Work out the finished part from the listing and answer in its coordinate system (mm). Give positions to 0.01 mm unless a question says otherwise; leave off trailing zeros. Loops run counter-clockwise (first coordinate to the right, second up) from the corner with the lowest first, then second, coordinate; pieces in that order, holes last. Notation, with made-up numbers: (28, -2) - (82, -2) arc R14 cw to (82, 24) - close; hole circle Ø7 at (-12.75, -20.75). An arc over 180 degrees is marked (long way). One line per question, with ' | ' between items. Start each with the question number.
1. Section C-C (y = -5.25) is taken. Determine the outline of the cut face in (x, z), plus the area to 3 significant figures.
2. Section A-A (x = 68) is taken. Determine the outline of the cut face in (y, z), plus the area to 3 significant figures.
3. Find the intervals of material crossed by line 1 (X direction, y = -10.25, z = 318.5); line 2 (Z direction, x = 124, y = -7); line 3 (Z direction, x = 54, y = -14), in increasing order.
4. Section B-B (z = 82) is taken. Determine the outline of the cut face in (x, y), plus the area to 3 significant figures.
from build123d import *

# Parameters (mm, degrees)
F0_W      = 28.8499742746
F0_H      = 37.8827601671
F1_DEPTH  = 16
F2_DEPTH  = 296
F3_DEPTH  = 996
F4_W      = 199.8313069344
F4_H      = 801.1276721954
F5_DEPTH  = 5
F6_DEPTH  = 39.21
F7_DEPTH  = 2.24
F8_DEPTH  = 55.66
F9_DEPTH  = 1.59
F10_W     = 54.77245152
F10_H     = 895.9976721954
F11_DEPTH = 5
F12_DEPTH = 5.86
F13_DEPTH = 18.91
F14_W     = 83.0026693535
F14_H     = 34.9487662315
F14_H_2   = 55.274695158
F15_W     = 82.9961860609
F15_H     = 44.8832511902
F15_H_2   = 52.5203943253
F16_DEPTH = 5
F17_DEPTH = 300
F18_DEPTH = 300
F19_DEPTH = 324.79
F20_DEPTH = 324.79
F21_DEPTH = 250
F22_DEPTH = 250
F23_DEPTH = 100
F24_DEPTH = 100
F25_DEPTH = 50
F26_DEPTH = 50
F27_DEPTH = 134.02
F28_DEPTH = 100
F29_DEPTH = 100
F30_DEPTH = 100
F31_DEPTH = 50
F32_DEPTH = 54.95
F33_DEPTH = 50
F34_DEPTH = 109.29
F35_DEPTH = 14.88
F36_DEPTH = 230.15
F37_DEPTH = 230.15
F38_DEPTH = 22.52
F39_DEPTH = 77.2
F40_DEPTH = 77.2
F41_DEPTH = 11
F42_R     = 3


with BuildPart() as f1:
    # F0 (on Front) → F1 (new body)
    with BuildSketch(Plane.XZ):
        with Locations((14.4249871373, 18.9413800836)):
            Rectangle(F0_W, F0_H)
    extrude(amount=F1_DEPTH)

    # F2 (add): a face of the model
    f2_faces = [f1.faces().sort_by_distance(p)[0] for p in [
        (0, -8, 18.9413800836),
    ]]
    extrude(f2_faces, amount=-F2_DEPTH)

    # F3 (add): a face of the model
    f3_faces = [f1.faces().sort_by_distance(p)[0] for p in [
        (148, -8, 0),
    ]]
    extrude(f3_faces, amount=-F3_DEPTH)

    # F4 (on face) → F5 (cut)
    with BuildSketch(Plane.XZ.offset(16)):
        with Locations((148.3252942562, 506.2239170074)):
            Rectangle(F4_W, F4_H)
    extrude(amount=-F5_DEPTH, mode=Mode.SUBTRACT)

    # F6 (cut): a face of the model
    f6_faces = [f1.faces().sort_by_distance(p)[0] for p in [
        (148.3252942562, -13.5, 906.7877531052),
    ]]
    extrude(f6_faces, amount=-F6_DEPTH, mode=Mode.SUBTRACT)

    # F7 (add): a face of the model
    f7_faces = [f1.faces().sort_by_distance(p)[0] for p in [
        (248.2409477234, -13.5, 525.8289170074),
    ]]
    extrude(f7_faces, amount=F7_DEPTH)

    # F8 (cut): a face of the model
    f8_faces = [f1.faces().sort_by_distance(p)[0] for p in [
        (147.2052942562, -13.5, 105.6600809097),
    ]]
    extrude(f8_faces, amount=-F8_DEPTH, mode=Mode.SUBTRACT)

    # F9 (add): a face of the model
    f9_faces = [f1.faces().sort_by_distance(p)[0] for p in [
        (48.409640789, -13.5, 497.9989170074),
    ]]
    extrude(f9_faces, amount=F9_DEPTH)

    # F10 (on face) → F11 (join)
    with BuildSketch(Plane.XZ.offset(11)):
        with Locations((154.5285359025, 497.9989170074)):
            Rectangle(F10_W, F10_H)
    extrude(amount=F11_DEPTH)

    # F12 (cut): a face of the model
    f12_faces = [f1.faces().sort_by_distance(p)[0] for p in [
        (127.1423101425, -13.5, 497.9989170074),
    ]]
    extrude(f12_faces, amount=-F12_DEPTH, mode=Mode.SUBTRACT)

    # F13 (cut): a face of the model
    f13_faces = [f1.faces().sort_by_distance(p)[0] for p in [
        (181.9147616625, -13.5, 497.9989170074),
    ]]
    extrude(f13_faces, amount=-F13_DEPTH, mode=Mode.SUBTRACT)

    # F14 (on face) + F15 (on face) → F16 (join)
    with BuildSketch(Plane.XZ.offset(11)):
        with Locations((91.5009754658, 853.3093035221)):
            Rectangle(F14_W, F14_H)
        with Locations((91.5009754658, 511.6568356752)):
            Rectangle(F14_W, F14_H_2)
    with BuildSketch(Plane.XZ.offset(11)):
        with Locations((204.5028546929, 853.7013530731)):
            Rectangle(F15_W, F15_H)
        with Locations((204.5028546929, 576.5425562859)):
            Rectangle(F15_W, F15_H_2)
    extrude(amount=F16_DEPTH)

    # F17 (add): faces of the model
    f17_faces = [f1.faces().sort_by_distance(p)[0] for p in [
        (204.5028546929, -13.5, 550.2823591232),
        (91.5009754658, -13.5, 484.0194880962),
    ]]
    extrude(f17_faces, amount=F17_DEPTH)

    # F18 (cut): faces of the model
    f18_faces = [f1.faces().sort_by_distance(p)[0] for p in [
        (91.5009754658, -13.5, 539.2941832542),
        (204.5028546929, -13.5, 602.8027534485),
    ]]
    extrude(f18_faces, amount=-F18_DEPTH, mode=Mode.SUBTRACT)

    # F19 (add): a face of the model
    f19_faces = [f1.faces().sort_by_distance(p)[0] for p in [
        (91.5009754658, -13.5, 835.8349204063),
    ]]
    extrude(f19_faces, amount=F19_DEPTH)

    # F20 (cut): a face of the model
    f20_faces = [f1.faces().sort_by_distance(p)[0] for p in [
        (91.5009754658, -13.5, 870.7836866379),
    ]]
    extrude(f20_faces, amount=-F20_DEPTH, mode=Mode.SUBTRACT)

    # F21 (add): a face of the model
    f21_faces = [f1.faces().sort_by_distance(p)[0] for p in [
        (91.5009754658, -13.5, 239.2941832542),
    ]]
    extrude(f21_faces, amount=F21_DEPTH)

    # F22 (cut): a face of the model
    f22_faces = [f1.faces().sort_by_distance(p)[0] for p in [
        (91.5009754658, -13.5, 184.0194880962),
    ]]
    extrude(f22_faces, amount=-F22_DEPTH, mode=Mode.SUBTRACT)

    # F23 (add): a face of the model
    f23_faces = [f1.faces().sort_by_distance(p)[0] for p in [
        (91.5009754658, -13.5, 545.9936866379),
    ]]
    extrude(f23_faces, amount=F23_DEPTH)

    # F24 (cut): a face of the model
    f24_faces = [f1.faces().sort_by_distance(p)[0] for p in [
        (91.5009754658, -13.5, 511.0449204063),
    ]]
    extrude(f24_faces, amount=-F24_DEPTH, mode=Mode.SUBTRACT)

    # F25 (add): a face of the model
    f25_faces = [f1.faces().sort_by_distance(p)[0] for p in [
        (91.5009754658, -13.5, 645.9936866379),
    ]]
    extrude(f25_faces, amount=F25_DEPTH)

    # F26 (cut): a face of the model
    f26_faces = [f1.faces().sort_by_distance(p)[0] for p in [
        (91.5009754658, -13.5, 611.0449204063),
    ]]
    extrude(f26_faces, amount=-F26_DEPTH, mode=Mode.SUBTRACT)

    # F27 (add): a face of the model
    f27_faces = [f1.faces().sort_by_distance(p)[0] for p in [
        (91.5009754658, -13.5, 434.0194880962),
    ]]
    extrude(f27_faces, amount=F27_DEPTH)

    # F28 (cut): a face of the model
    f28_faces = [f1.faces().sort_by_distance(p)[0] for p in [
        (91.5009754658, -13.5, 299.9994880962),
    ]]
    extrude(f28_faces, amount=-F28_DEPTH, mode=Mode.SUBTRACT)

    # F29 (add): a face of the model
    f29_faces = [f1.faces().sort_by_distance(p)[0] for p in [
        (91.5009754658, -13.5, 661.0449204063),
    ]]
    extrude(f29_faces, amount=F29_DEPTH)

    # F30 (cut): a face of the model
    f30_faces = [f1.faces().sort_by_distance(p)[0] for p in [
        (91.5009754658, -13.5, 695.9936866379),
    ]]
    extrude(f30_faces, amount=-F30_DEPTH, mode=Mode.SUBTRACT)

    # F31 (add): a face of the model
    f31_faces = [f1.faces().sort_by_distance(p)[0] for p in [
        (91.5009754658, -13.5, 595.9936866379),
    ]]
    extrude(f31_faces, amount=F31_DEPTH)

    # F32 (cut): a face of the model
    f32_faces = [f1.faces().sort_by_distance(p)[0] for p in [
        (91.5009754658, -13.5, 561.0449204063),
    ]]
    extrude(f32_faces, amount=-F32_DEPTH, mode=Mode.SUBTRACT)

    # F33 (add): a face of the model
    f33_faces = [f1.faces().sort_by_distance(p)[0] for p in [
        (91.5009754658, -13.5, 399.9994880962),
    ]]
    extrude(f33_faces, amount=F33_DEPTH)

    # F34 (cut): a face of the model
    f34_faces = [f1.faces().sort_by_distance(p)[0] for p in [
        (91.5009754658, -13.5, 489.2941832542),
    ]]
    extrude(f34_faces, amount=-F34_DEPTH, mode=Mode.SUBTRACT)

    # F35 (cut): a face of the model
    f35_faces = [f1.faces().sort_by_distance(p)[0] for p in [
        (204.5028546929, -13.5, 831.259727478),
    ]]
    extrude(f35_faces, amount=-F35_DEPTH, mode=Mode.SUBTRACT)

    # F36 (add): a face of the model
    f36_faces = [f1.faces().sort_by_distance(p)[0] for p in [
        (204.5028546929, -13.5, 846.139727478),
    ]]
    extrude(f36_faces, amount=F36_DEPTH)

    # F37 (cut): a face of the model
    f37_faces = [f1.faces().sort_by_distance(p)[0] for p in [
        (204.5028546929, -13.5, 876.1429786682),
    ]]
    extrude(f37_faces, amount=-F37_DEPTH, mode=Mode.SUBTRACT)

    # F38 (cut): a face of the model
    f38_faces = [f1.faces().sort_by_distance(p)[0] for p in [
        (204.5028546929, -13.5, 250.2823591232),
    ]]
    extrude(f38_faces, amount=-F38_DEPTH, mode=Mode.SUBTRACT)

    # F39 (add): a face of the model
    f39_faces = [f1.faces().sort_by_distance(p)[0] for p in [
        (204.5028546929, -13.5, 302.8027534485),
    ]]
    extrude(f39_faces, amount=F39_DEPTH)

    # F40 (cut): a face of the model
    f40_faces = [f1.faces().sort_by_distance(p)[0] for p in [
        (204.5028546929, -13.5, 272.8023591232),
    ]]
    extrude(f40_faces, amount=-F40_DEPTH, mode=Mode.SUBTRACT)

    # F41 (cut): faces of the model
    f41_faces = [f1.faces().sort_by_distance(p)[0] for p in [
        (91.5009754658, -11, 795.9957198715),
        (204.5028546929, -11, 795.9953658867),
        (204.5028546929, -11, 497.9962404633),
        (91.5009754658, -11, 497.9995518303),
        (91.5009754658, -11, 199.999784503),
        (204.5028546929, -11, 200.0012200165),
    ]]
    extrude(f41_faces, amount=-F41_DEPTH, mode=Mode.SUBTRACT)

    # F42
    f42_edges = [f1.edges().sort_by_distance(p)[0] for p in [
        (0, -16, 498),
        (148, -16, 0),
        (296, -16, 498),
        (148, -16, 996),
        (133.00231, -16, 199.999785),
        (91.500975, -16, 50.000081),
        (49.999641, -16, 199.999785),
        (91.500975, -16, 349.999488),
        (246.000948, -16, 200.00122),
        (204.502855, -16, 50.000081),
        (163.004762, -16, 200.00122),
        (204.502855, -16, 350.002359),
        (163.004762, -16, 497.99624),
        (204.502855, -16, 615.989727),
        (246.000948, -16, 497.99624),
        (204.502855, -16, 380.002753),
        (91.500975, -16, 615.99492),
        (133.00231, -16, 497.999552),
        (91.500975, -16, 380.004183),
        (49.999641, -16, 497.999552),
        (49.999641, -16, 795.99572),
        (91.500975, -16, 945.997753),
        (133.00231, -16, 795.99572),
        (91.500975, -16, 645.993687),
        (163.004762, -16, 795.995366),
        (204.502855, -16, 945.997753),
        (246.000948, -16, 795.995366),
        (204.502855, -16, 645.992979),
    ]]
    fillet(f42_edges, radius=F42_R)


solid = f1.part
Conclusion:
1) outline: (0, 0) - (296, 0) - (296, 996) - (0, 996) - close; hole (50, 50) - (133, 50) - (133, 350) - (50, 350) - close; hole (50, 380) - (133, 380) - (133, 615.99) - (50, 615.99) - close; hole (50, 645.99) - (133, 645.99) - (133, 946) - (50, 946) - close; hole (163, 50) - (246, 50) - (246, 350) - (163, 350) - close; hole (163, 380) - (246, 380) - (246, 615.99) - (163, 615.99) - close; hole (163, 645.99) - (246, 645.99) - (246, 946) - (163, 946) - close | area: 156,000 mm²
2) outline: (-16, 3) arc R3 ccw to (-13, 0) - (0, 0) - (0, 50) - (-13, 50) arc R3 ccw to (-16, 47) - close; (-16, 353) arc R3 ccw to (-13, 350) - (0, 350) - (0, 380) - (-13, 380) arc R3 ccw to (-16, 377) - close; (-16, 618.99) arc R3 ccw to (-13, 615.99) - (0, 615.99) - (0, 645.99) - (-13, 645.99) arc R3 ccw to (-16, 642.99) - close; (-16, 949) arc R3 ccw to (-13, 946) - (0, 946) - (0, 996) - (-13, 996) arc R3 ccw to (-16, 993) - close | area: 2,540 mm²
3) line 1: 0 to 50, 133 to 163, 246 to 296 | line 2: 0 to 50, 350 to 380, 615.99 to 645.99, 946 to 996 | line 3: 0.17 to 49.83, 350.17 to 379.83, 616.17 to 645.82, 946.17 to 995.83
4) outline: (0, -13) arc R3 ccw to (3, -16) - (47, -16) arc R3 ccw to (50, -13) - (50, 0) - (0, 0) - close; (133, -13) arc R3 ccw to (136, -16) - (160, -16) arc R3 ccw to (163, -13) - (163, 0) - (133, 0) - close; (246, -13) arc R3 ccw to (249, -16) - (293, -16) arc R3 ccw to (296, -13) - (296, 0) - (246, 0) - close | area: 2,070 mm²
